```python
from build123d import *

# Parameters (mm, degrees)
ESQUISSE3_W             = 190
ESQUISSE3_H             = 146
BOSS_EXTRU_3_DEPTH      = 3
ESQUISSE4_W             = 190
ESQUISSE4_H             = 3
BOSS_EXTRU_4_DEPTH      = 75
ESQUISSE5_W             = 190
ESQUISSE5_H             = 3
BOSS_EXTRU_5_DEPTH      = 75
ESQUISSE6_W             = 3
ESQUISSE6_H             = 140
BOSS_EXTRU_6_DEPTH      = 75
ESQUISSE7_W             = 3
ESQUISSE7_H             = 140
BOSS_EXTRU_7_DEPTH      = 75
ESQUISSE8_W             = 26
ESQUISSE8_H             = 140
ENL_V_MAT_EXTRU_1_DEPTH = 5
ESQUISSE9_W             = 50
ESQUISSE9_H             = 13.580457403
BOSS_EXTRU_8_DEPTH      = 30
ESQUISSE10_W            = 5
ESQUISSE10_H            = 126.419542597
BOSS_EXTRU_9_DEPTH      = 30
ESQUISSE12_W            = 45
ESQUISSE12_H            = 116.062132341
BOSS_EXTRU_10_DEPTH     = 5
ESQUISSE13_W            = 137
ESQUISSE13_H            = 5
BOSS_EXTRU_11_DEPTH     = 30
ESQUISSE14_W            = 134
ESQUISSE14_H            = 10
BOSS_EXTRU_12_DEPTH     = 4
ESQUISSE15_W            = 26
ESQUISSE15_H            = 10
BOSS_EXTRU_13_DEPTH     = 5
ESQUISSE16_W            = 4
ESQUISSE16_H            = 125
BOSS_EXTRU_14_DEPTH     = 7
ESQUISSE17_W            = 22.881021534
ESQUISSE17_H            = 72.322375242
ENL_V_MAT_EXTRU_2_DEPTH = 3
ESQUISSE19_W            = 44.999866494
ESQUISSE19_H            = 10.48475091
BOSS_EXTRU_15_DEPTH     = 3


with BuildPart() as part:
    # Esquisse3 → Boss.-Extru.3 (new body)
    with BuildSketch(Plane.XY):
        Rectangle(ESQUISSE3_W, ESQUISSE3_H)
    extrude(amount=BOSS_EXTRU_3_DEPTH)

    # Esquisse4 → Boss.-Extru.4 (add)
    with BuildSketch(Plane(origin=(0, 0, 0), x_dir=(-1, 0, 0), z_dir=(0, 0, -1))):
        with Locations((0, -71.5)):
            Rectangle(ESQUISSE4_W, ESQUISSE4_H)
    extrude(amount=BOSS_EXTRU_4_DEPTH)

    # Esquisse5 → Boss.-Extru.5 (add)
    with BuildSketch(Plane(origin=(0, 0, 0), x_dir=(-1, 0, 0), z_dir=(0, 0, -1))):
        with Locations((0, 71.5)):
            Rectangle(ESQUISSE5_W, ESQUISSE5_H)
    extrude(amount=BOSS_EXTRU_5_DEPTH)

    # Esquisse6 → Boss.-Extru.6 (add)
    with BuildSketch(Plane(origin=(0, 0, 0), x_dir=(-1, 0, 0), z_dir=(0, 0, -1))):
        with Locations((93.5, 0)):
            Rectangle(ESQUISSE6_W, ESQUISSE6_H)
    extrude(amount=BOSS_EXTRU_6_DEPTH)

    # Esquisse7 → Boss.-Extru.7 (add)
    with BuildSketch(Plane(origin=(0, 0, 0), x_dir=(-1, 0, 0), z_dir=(0, 0, -1))):
        with Locations((-93.5, 0)):
            Rectangle(ESQUISSE7_W, ESQUISSE7_H)
    extrude(amount=BOSS_EXTRU_7_DEPTH)

    # Esquisse8 → Enlèv. mat.-Extru.1 (cut)
    with BuildSketch(Plane.ZY.offset(-92)):
        with Locations((-13, 0)):
            Rectangle(ESQUISSE8_W, ESQUISSE8_H)
    extrude(amount=-ENL_V_MAT_EXTRU_1_DEPTH, mode=Mode.SUBTRACT)

    # Esquisse9 → Boss.-Extru.8 (add)
    with BuildSketch(Plane(origin=(0, 0, 0), x_dir=(-1, 0, 0), z_dir=(0, 0, -1))):
        with Locations((67, 63.209771299)):
            Rectangle(ESQUISSE9_W, ESQUISSE9_H)
    extrude(amount=BOSS_EXTRU_8_DEPTH)

    # Esquisse10 → Boss.-Extru.9 (add)
    with BuildSketch(Plane(origin=(0, 0, 0), x_dir=(-1, 0, 0), z_dir=(0, 0, -1))):
        with Locations((44.5, -6.790228701)):
            Rectangle(ESQUISSE10_W, ESQUISSE10_H)
    extrude(amount=BOSS_EXTRU_9_DEPTH)

    # Esquisse12 → Boss.-Extru.10 (add)
    with BuildSketch(Plane(origin=(0, 0, -30), x_dir=(-1, 0, 0), z_dir=(0, 0, -1))):
        with Locations((69.5, -1.611523574)):
            Rectangle(ESQUISSE12_W, ESQUISSE12_H)
    extrude(amount=-BOSS_EXTRU_10_DEPTH)

    # Esquisse13 → Boss.-Extru.11 (add)
    with BuildSketch(Plane(origin=(0, 0, 0), x_dir=(-1, 0, 0), z_dir=(0, 0, -1))):
        with Locations((-26.5, -57.5)):
            Rectangle(ESQUISSE13_W, ESQUISSE13_H)
    extrude(amount=BOSS_EXTRU_11_DEPTH)

    # Esquisse14 → Boss.-Extru.12 (add)
    with BuildSketch(Plane(origin=(0, 0, -30), x_dir=(-1, 0, 0), z_dir=(0, 0, -1))):
        with Locations((-25, -65)):
            Rectangle(ESQUISSE14_W, ESQUISSE14_H)
    extrude(amount=-BOSS_EXTRU_12_DEPTH)

    # Esquisse15 → Boss.-Extru.13 (add)
    with BuildSketch(Plane(origin=(95, 0, 0), x_dir=(0, 0, -1), z_dir=(1, 0, 0))):
        with Locations((13, -65)):
            Rectangle(ESQUISSE15_W, ESQUISSE15_H)
    extrude(amount=-BOSS_EXTRU_13_DEPTH)

    # Esquisse16 → Boss.-Extru.14 (add)
    with BuildSketch(Plane.ZY.offset(-92)):
        with Locations((-28, 7.5)):
            Rectangle(ESQUISSE16_W, ESQUISSE16_H)
    extrude(amount=BOSS_EXTRU_14_DEPTH)

    # Esquisse17 → Enlèv. mat.-Extru.2 (cut)
    with BuildSketch(Plane.ZY.offset(-92)):
        with Locations((-41.440510767, 33.838812379)):
            Rectangle(ESQUISSE17_W, ESQUISSE17_H)
    extrude(amount=-ENL_V_MAT_EXTRU_2_DEPTH, mode=Mode.SUBTRACT)

    # Esquisse19 → Boss.-Extru.15 (add)
    with BuildSketch(Plane(origin=(0, 0, -30), x_dir=(-1, 0, 0), z_dir=(0, 0, -1))):
        with Locations((69.499933247, -64.884965199)):
            Rectangle(ESQUISSE19_W, ESQUISSE19_H)
    extrude(amount=-BOSS_EXTRU_15_DEPTH)


solid = part.part
```
Check sheet for the modelled part. Datum: model origin and axes. Units: mm. A direction names the side the tool comes from. Give positions to 0.01 mm unless a question says otherwise; leave off trailing zeros. Write each loop counter-clockwise with the first axis right and the second up, starting at its lowest first coordinate (ties: lowest second). Pieces come first, ordered by that corner, then holes.
Item 1: Cross-section at D-D (y = -44.5). Enter the section's corners in (x, z), and give its area (4 significant figures).
Item 2: Cross-section at B-B (z = -56.5). Enter the section's corners in (x, y), and give its area (3 significant figures).
Item 3: Cross-section at C-C (x = 73). Enter the section's corners in (y, z).
Item 4: Gauge pin test, flat ends, axial feed: pin 1 (8 mm diameter, centred on x = -6, y = -66.5, fed in from -Z); pin 2 (10 mm diameter, centred on x = -62, y = -22.5, fed in from -Z); pin 3 (10 mm diameter, centred on x = 34, y = 28.5, fed in from -Z). Record the tip position at first contact, or that the pin passes through.
Item 5: Cross-section at A-A (y = 29.5). Enter the section's corners in (x, z), and give its area (3 significant figures).
Item 6: Draft check along X on faces 3 (the face through (26, 7, 0)), 4 (the face through (-95, -1, -35)), 5 (the face through (23, -65, 0)). Enter one of: released by +X, released by -X, zero draft, split by the parting line, or undercut.
Item 7: Access from +Z, -Z, +X, -X, +Y, -Y to the whole of each face (thin tool, end or side, straight path). Record for faces 1 (the face through (-1, 1, 3)), 2 (the face through (-47, -8, -13)).
Item 8: Scan lines: L1, parallel to Y at x = -22, z = -20; L2, parallel to X at y = -58.5, z = -49; L3, parallel to X at y = 3, z = -1.5. Record each from-to range of solid material in increasing order.
Report:
1. outline: (-95, -75) - (-92, -75) - (-92, -30) - (-42, -30) - (-42, 0) - (95, 0) - (95, 3) - (-95, 3) - close; (85, -30) - (92, -30) - (92, -75) - (95, -75) - (95, -26) - (85, -26) - close; hole (-92, -25) - (-47, -25) - (-47, 0) - (-92, 0) - close
1. area: 1,345 mm2
2. outline: (-95, -73) - (95, -73) - (95, 73) - (-95, 73) - close; hole (-92, -70) - (92, -70) - (92, 70) - (-92, 70) - close
2. area: 1,980 mm2
3. outline: (-73, -75) - (-70, -75) - (-70, -30) - (-55, -30) - (-55, 0) - (70, 0) - (70, -75) - (73, -75) - (73, 3) - (-73, 3) - close; hole (-70, -26) - (-60, -26) - (-60, 0) - (-70, 0) - close
4. pin 1: stops at z = -75
4. pin 2: stops at z = -30
4. pin 3: stops at z = 0
5. outline: (-95, -75) - (-92, -75) - (-92, -30) - (-42, -30) - (-42, 0) - (95, 0) - (95, 3) - (-95, 3) - close; (85, -30) - (95, -30) - (95, -26) - (85, -26) - close; (92, -75) - (95, -75) - (95, -52.88) - (92, -52.88) - close; hole (-92, -25) - (-47, -25) - (-47, 0) - (-92, 0) - close
5. area: 1,280 mm2
6. face 3: zero draft
6. face 4: released by -X
6. face 5: undercut
7. face 1: +Z, +X, -X, +Y, -Y
7. face 2: none
8. L1: y = -73 to -70, -60 to -55, 70 to 73
8. L2: x = -95 to -92, 92 to 95
8. L3: x = -95 to -92, -47 to -42
